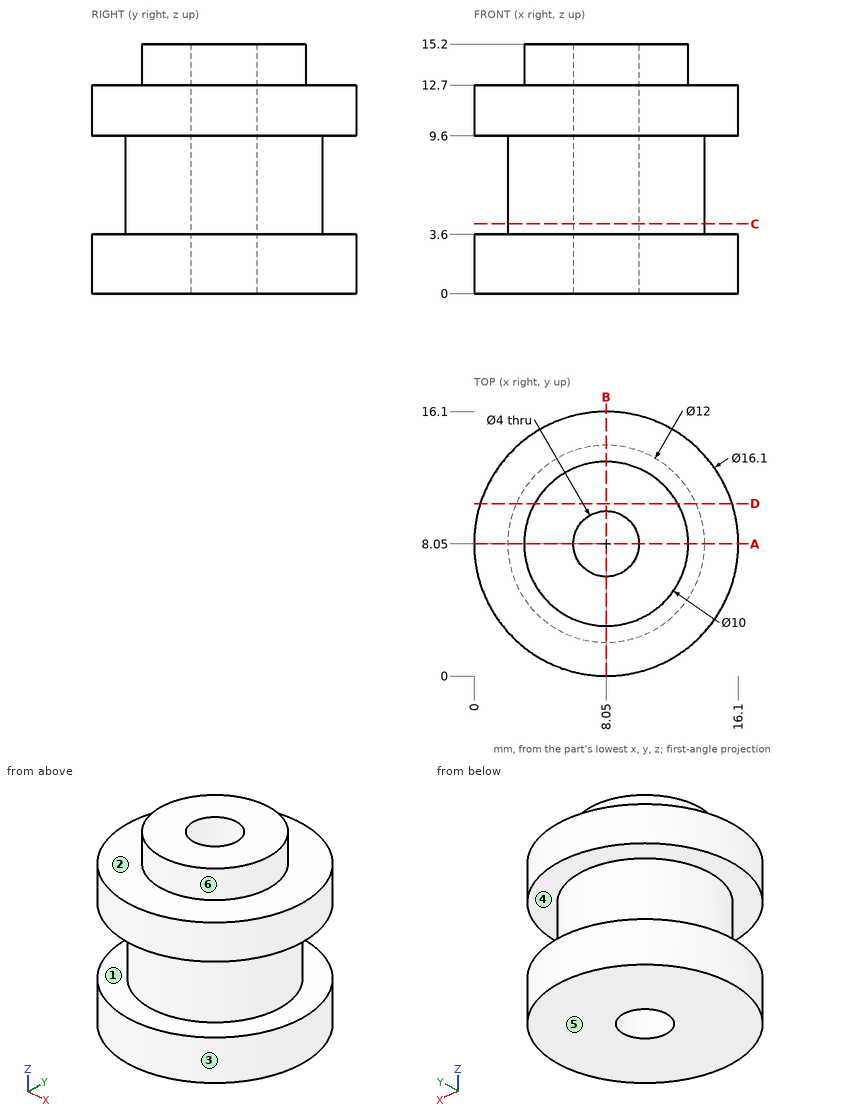
Design review of the part shown in the three views and the two pictorial views. Dimensions are in mm from the part's minimum x, y and z. A direction names the side the tool comes from. Give positions to 0.01 mm unless a question says otherwise; leave off trailing zeros. Loops run counter-clockwise (first coordinate to the right, second up) from the corner with the lowest first, then second, coordinate; pieces in that order, holes last. Notation, with made-up numbers: (64.5, -8.75) - (100.5, -8.75) arc R33 ccw to (100.5, 25.25) - close; hole circle Ø6 at (-12.5, -30). An arc over 180 degrees is marked (long way). Write item = value, one per line.
1) To check wall thickness, follow line 1 (Z direction, x = 15.25, y = 10.75); line 2 (Y direction, x = 8.05, z = 10.25); line 3 (Y direction, x = 8.05, z = 4). State the ranges of each line that lie inside material, in increasing order.
Result sheet:
line_1 = 0 to 3.6, 9.6 to 12.7
line_2 = 0 to 6.05, 10.05 to 16.1
line_3 = 2.05 to 6.05, 10.05 to 14.05
2) Clearance check with flat-ended pins moving along their axes: pin 1 Ø1.5 at (x, z) = (3.5, 6) entering from -Y; pin 2 Ø3 at (x, z) = (13.5, 4) entering from -Y; pin 3 Ø1.5 at (x, z) = (4.5, 11.5) entering from +Y. State where each tip first meets the part, or that it passes through.
Result sheet:
pin_1 = 3.41
pin_2 = 1.07
pin_3 = 15.6
3) Tool access review of the marked faces 1, 2 and 3: name each direction out of +Z, -Z, +X, -X, +Y, -Y from which nothing blocks a thin tool from reaching the whole face with its end or side.
Result sheet:
face_1 = none
face_2 = +Z
face_3 = +Z, -Z
4) Take a section at C-C on z = 4.25. State the section outline as (x, y) points.
Result sheet:
outline = circle Ø12 at (8.05, 8.05); hole circle Ø4 at (8.05, 8.05)
5) Take a section at A-A on y = 8.05. State the section outline as (x, z) points, and give its area (3 significant figures).
Result sheet:
outline = (0, 0) - (6.05, 0) - (6.05, 15.2) - (3.05, 15.2) - (3.05, 12.7) - (0, 12.7) - (0, 9.6) - (2.05, 9.6) - (2.05, 3.6) - (0, 3.6) - close; (10.05, 0) - (16.1, 0) - (16.1, 3.6) - (14.05, 3.6) - (14.05, 9.6) - (16.1, 9.6) - (16.1, 12.7) - (13.05, 12.7) - (13.05, 15.2) - (10.05, 15.2) - close
area = 144 mm2
6) Draft analysis for pull direction Z (two halves, no side actions). For the marked faces 4, 5 and 6, state which applies: +Z half, -Z half, draft (parallel to the pull), parting line (faces both ways), or undercut.
Result sheet:
face_4 = undercut
face_5 = -Z half
face_6 = draft
7) Take a section at D-D on y = 10.5. State the section outline as (x, z) points.
Result sheet:
outline = (0.38, 0) - (15.72, 0) - (15.72, 3.6) - (13.53, 3.6) - (13.53, 9.6) - (15.72, 9.6) - (15.72, 12.7) - (12.41, 12.7) - (12.41, 15.2) - (3.69, 15.2) - (3.69, 12.7) - (0.38, 12.7) - (0.38, 9.6) - (2.57, 9.6) - (2.57, 3.6) - (0.38, 3.6) - close
